```python
from build123d import *

# Parameters (mm, degrees)
SKETCH2_W           = 100
SKETCH2_H           = 147
SKETCH2_W_2         = 40
SKETCH2_H_2         = 20
BOSS_EXTRUDE1_DEPTH = 4.5


with BuildPart() as part:
    # Sketch2 → Boss-Extrude1 (new body)
    with BuildSketch(Plane(origin=(0, 0, 0), x_dir=(1, 0, 0), z_dir=(0, 1, 0))):
        with Locations((0, -2.47075608)):
            Rectangle(SKETCH2_W, SKETCH2_H)
        with Locations((0, 29.02924392)):
            Rectangle(SKETCH2_W_2, SKETCH2_H_2, mode=Mode.SUBTRACT)
        Polygon((-45, -6.97075608), (-30, -6.97075608), (-30, -9.97075608), (-40, -9.97075608), (-40, -16.47075608), (-30, -16.47075608), (-30, -19.47075608), (-45, -19.47075608), (-45, -16.47075608), (-43, -16.47075608), (-43, -9.97075608), (-45, -9.97075608), align=None, mode=Mode.SUBTRACT)
        Polygon((43, -9.97075608), (45, -9.97075608), (45, -6.97075608), (30, -6.97075608), (30, -9.97075608), (40, -9.97075608), (40, -16.47075608), (30, -16.47075608), (30, -19.47075608), (45, -19.47075608), (45, -16.47075608), (43, -16.47075608), align=None, mode=Mode.SUBTRACT)
    extrude(amount=BOSS_EXTRUDE1_DEPTH)


solid = part.part
```
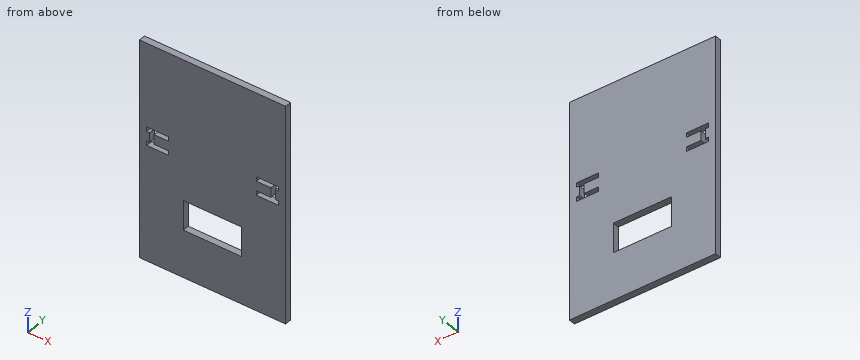
Verification items for the finished model (mm, model axes). Give positions to 0.01 mm unless a question says otherwise; leave off trailing zeros. Order: outer loops, then holes, each group sorted by start corner. A loop starts at its lowest first (then second) coordinate and runs counter-clockwise, first axis right, second up. Notation, with made-up numbers: M -6,29 L 37,29 A12 cw 37,45 Z; hole C 56,77 d3. An arc over 180 degrees is marked long. Return JSON: item names as keys, results as strings. Group by question number.
1) Section check C-C on x = -12. Record the cut outline in (y, z).
2) Go/stop test with a flat-tipped pin: pin 1 Ø1 at (x, z) = (-31.5, 6.5) entering from -Y. Record where the tip stops, or that it passes through.
3) Section check A-A on x = 32. Record the cut outline in (y, z).
4) Section check B-B on z = -34. Record the cut outline in (x, y).
5) Scan lines: line 1 (Z direction, x = 31, y = 0.7); line 2 (Z direction, x = 2, y = 3.65); line 3 (X direction, y = 1.4, z = -28). Record each from-to range of solid material in increasing order.
6) Section check D-D on y = 3.05. Give the number of separate pieces and of enclosed holes in the cut face, and give its area (3 significant figures).
Answer block:
{
 "1": {"outline": "M 0,-71.03 L 4.5,-71.03 L 4.5,-39.03 L 0,-39.03 Z; M 0,-19.03 L 4.5,-19.03 L 4.5,75.97 L 0,75.97 Z"},
 "2": {"pin 1": "stops at y = 0"},
 "3": {"outline": "M 0,-71.03 L 4.5,-71.03 L 4.5,6.97 L 0,6.97 Z; M 0,9.97 L 4.5,9.97 L 4.5,16.47 L 0,16.47 Z; M 0,19.47 L 4.5,19.47 L 4.5,75.97 L 0,75.97 Z"},
 "4": {"outline": "M -50,0 L -20,0 L -20,4.5 L -50,4.5 Z; M 20,0 L 50,0 L 50,4.5 L 20,4.5 Z"},
 "5": {"line 1": "z = -71.03 to 6.97, 9.97 to 16.47, 19.47 to 75.97", "line 2": "z = -71.03 to -39.03, -19.03 to 75.97", "line 3": "x = -50 to -20, 20 to 50"},
 "6": {"separate pieces": "1", "enclosed holes": "3", "area": "13,700 mm^2"}
}
